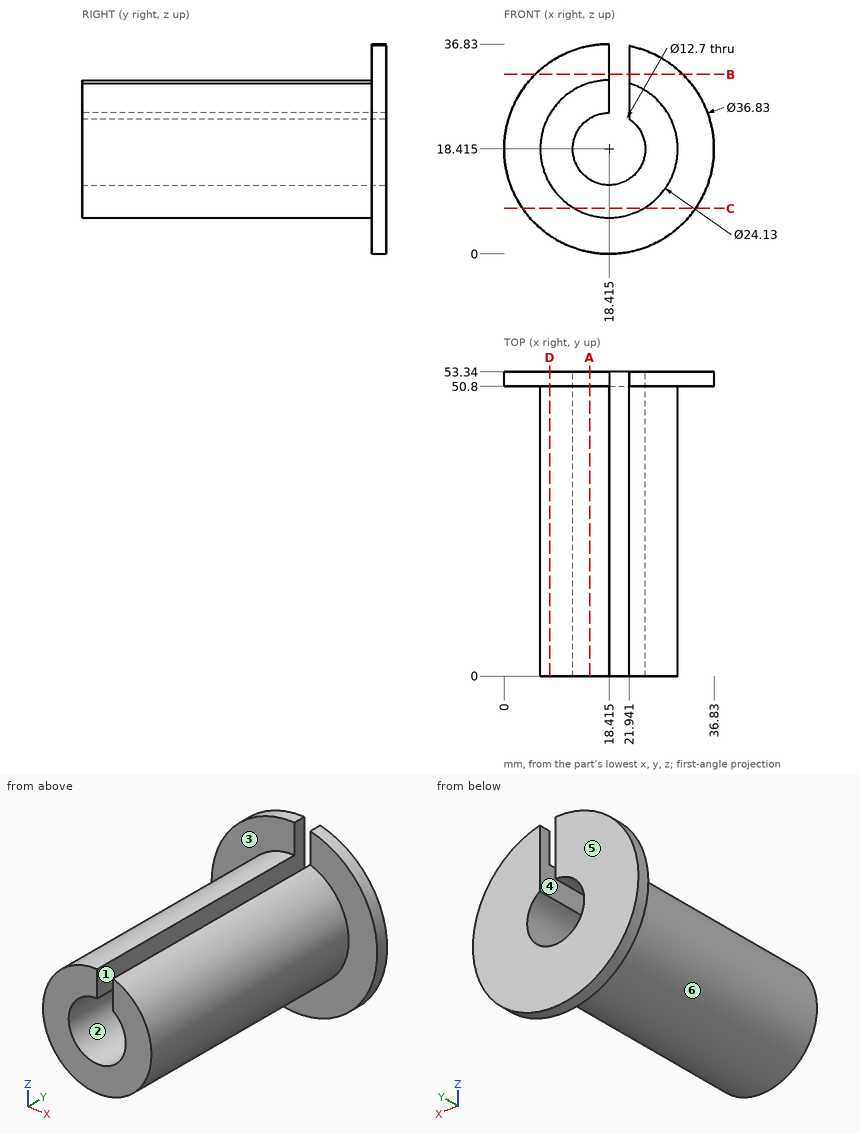
Answer from the drawing. Dimensions are ordinates in mm from the lowest x, y and z of the part. A direction names the side the tool comes from. Give positions to 0.01 mm unless a question says otherwise; leave off trailing zeros. Write each loop counter-clockwise with the first axis right and the second up, starting at its lowest first coordinate (ties: lowest second). Pieces come first, ordered by that corner, then holes. Notation, with made-up numbers: (47.25, 1.5) - (72.25, 1.5) arc R17 ccw to (72.25, 9.5) - close; hole circle Ø10 at (57.5, 65.25). An arc over 180 degrees is marked (long way). One line per item, written item: value. Start each with the question number.
1. Consider probe 1 along Y at (x, z) = (32, 17.5); probe 2 along X at (y, z) = (24, 13.5) (1 decimal); probe 3 along Z at (x, y) = (23, 26.5) (1 decimal). Determine where each line is inside the solid, lowest interval first.
2. Find section C-C (z = 8). Write down the section's boundary in (x, y) (1 decimal), then the cut area to 3 significant figures.
3. Find section A-A (x = 15). Write down the section's boundary in (y, z).
4. Find section B-B (z = 31.5). Write down the section's boundary in (x, y) (1 decimal).
5. For the marked faces 1, 2 and 3, determine the directions among +Z, -Z, +X, -X, +Y, -Y from which every point of the face is accessible in a straight line to the end or side of a thin tool.
6. Given pin 1 (1.5 mm diameter, centred on x = 33, y = 19, fed in from +Z); pin 2 (12 mm diameter, centred on y = 33, z = 12.5, fed in from +X); pin 3 (6 mm diameter, centred on x = 12, y = 32.5, fed in from -Z); pin 4 (6.5 mm diameter, centred on y = 13.5, z = 32, fed in from -X), each flat-ended and moving along its own axis, determine where each tip first touches the part or whether it passes through.
7. Find section D-D (x = 8). Write down the section's boundary in (y, z) (1 decimal).
8. For a pull along X with two mould halves and no side action, classify the marked faces 4, 5 and 6 as +X half, -X half, draft (parallel to the pull), parting line (faces both ways), or undercut.
Geometry results:
1. probe 1: 50.8 to 53.34
1. probe 2: 7.4 to 14.4, 22.4 to 29.4
1. probe 3: 7.3 to 14, 22.8 to 29.6
2. outline: (3.2, 50.8) - (12.3, 50.8) - (12.3, 0) - (24.5, 0) - (24.5, 50.8) - (33.6, 50.8) - (33.6, 53.3) - (3.2, 53.3) - close
2. area: 696 mm2
3. outline: (0, 6.84) - (50.8, 6.84) - (50.8, 0.32) - (53.34, 0.32) - (53.34, 13.06) - (0, 13.06) - close; (0, 23.77) - (53.34, 23.77) - (53.34, 36.51) - (50.8, 36.51) - (50.8, 29.99) - (0, 29.99) - close
4. outline: (5.5, 50.8) - (18.4, 50.8) - (18.4, 53.3) - (5.5, 53.3) - close; (21.9, 50.8) - (31.4, 50.8) - (31.4, 53.3) - (21.9, 53.3) - close
5. face 1: +Z, +Y, -Y
5. face 2: +Y, -Y
5. face 3: -Y
6. pin 1: through
6. pin 2: x = 30.48
6. pin 3: z = 6.84
6. pin 4: x = 12.19
7. outline: (0, 12.3) - (50.8, 12.3) - (50.8, 3.2) - (53.3, 3.2) - (53.3, 33.6) - (50.8, 33.6) - (50.8, 24.5) - (0, 24.5) - close
8. face 4: undercut
8. face 5: draft
8. face 6: parting line
